```python
from build123d import *

# Parameters (mm, degrees)
SKETCH1_W           = 330
SKETCH1_H           = 250
BOSS_EXTRUDE1_DEPTH = 6.9
SKETCH2_R           = 3
CUT_EXTRUDE1_DEPTH  = 7.9
SKETCH3_R           = 25
CUT_EXTRUDE2_DEPTH  = 7.9
FILLET1_R           = 20


with BuildPart() as part:
    # Sketch1 → Boss-Extrude1 (new body)
    with BuildSketch(Plane(origin=(0, 0, 0), x_dir=(1, 0, 0), z_dir=(0, 1, 0))):
        Rectangle(SKETCH1_W, SKETCH1_H)
    extrude(amount=BOSS_EXTRUDE1_DEPTH)

    # Sketch2 → Cut-Extrude1 (cut, through all)
    with BuildSketch(Plane(origin=(0, 6.9, 0), x_dir=(1, 0, 0), z_dir=(0, 1, 0))):
        with Locations((-145, 105)):
            Circle(SKETCH2_R)
        with Locations((145, 105)):
            Circle(SKETCH2_R)
        with Locations((145, -105)):
            Circle(SKETCH2_R)
        with Locations((-145, -105)):
            Circle(SKETCH2_R)
    extrude(amount=-CUT_EXTRUDE1_DEPTH, mode=Mode.SUBTRACT)

    # Sketch3 → Cut-Extrude2 (cut, through all)
    with BuildSketch(Plane(origin=(0, 6.9, 0), x_dir=(1, 0, 0), z_dir=(0, 1, 0))):
        Circle(SKETCH3_R)
    extrude(amount=-CUT_EXTRUDE2_DEPTH, mode=Mode.SUBTRACT)

    # Fillet1
    fillet1_edges = [part.edges().sort_by_distance(p)[0] for p in [
        (-165, 3.45, -125),
        (165, 3.45, -125),
        (165, 3.45, 125),
        (-165, 3.45, 125),
    ]]
    fillet(fillet1_edges, radius=FILLET1_R)


solid = part.part
```
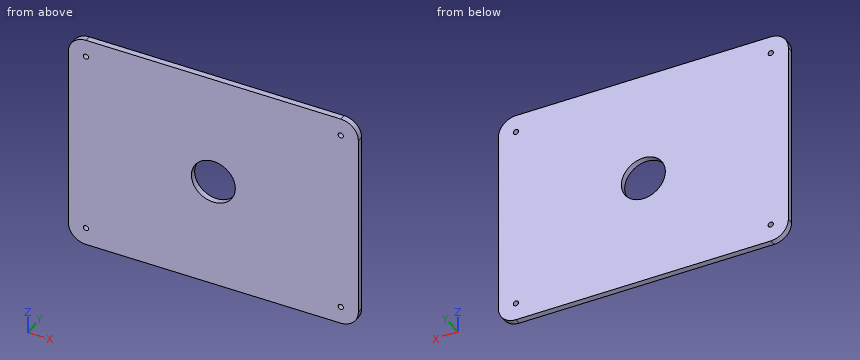
Input: part model. Units: mm. Frame: model coordinates. Round coordinates to 2 decimals unless told otherwise and drop trailing zeros. Write each loop counter-clockwise with the first axis right and the second up, starting at its lowest first coordinate (ties: lowest second). Pieces come first, ordered by that corner, then holes. Notation, with made-up numbers: (33.5, 15.25) - (72.5, 15.25) arc R10 ccw to (72.5, 30.25) - close; hole circle Ø4 at (38.5, 48.5). An arc over 180 degrees is marked (long way). Write item = value, one per line.
(1) Material intervals for probe 1 along X at (y, z) = (4.5, 105); probe 2 along Z at (x, y) = (-145, 5.75); probe 3 along X at (y, z) = (1.75, 0), sorted ascending.
Geometry check:
probe_1 = -165 to -148, -142 to 142, 148 to 165
probe_2 = -125 to -108, -102 to 102, 108 to 125
probe_3 = -165 to -25, 25 to 165
(2) Section query B-B on y = 4. Output: boundary loops of the cut face in (x, z), then the cut area to 3 significant figures.
Geometry check:
outline = (-165, -105) arc R20 ccw to (-145, -125) - (145, -125) arc R20 ccw to (165, -105) - (165, 105) arc R20 ccw to (145, 125) - (-145, 125) arc R20 ccw to (-165, 105) - close; hole circle Ø6 at (-145, -105); hole circle Ø6 at (-145, 105); hole circle Ø50 at (0, 0); hole circle Ø6 at (145, -105); hole circle Ø6 at (145, 105)
area = 80,100 mm^2
(3) Section query A-A on x = 0. Output: boundary loops of the cut face in (y, z).
Geometry check:
outline = (0, -125) - (6.9, -125) - (6.9, -25) - (0, -25) - close; (0, 25) - (6.9, 25) - (6.9, 125) - (0, 125) - close
(4) Section query C-C on z = 0. Output: boundary loops of the cut face in (x, y).
Geometry check:
outline = (-165, 0) - (-25, 0) - (-25, 6.9) - (-165, 6.9) - close; (25, 0) - (165, 0) - (165, 6.9) - (25, 6.9) - close
